For this review, take the finished solid that the model builds, in its own axes (mm). A direction names the side the tool comes from. Coordinates: 2 decimals unless noted, no trailing zeros. Write each loop counter-clockwise with the first axis right and the second up, starting at its lowest first coordinate (ties: lowest second). Pieces come first, ordered by that corner, then holes.
1) We need section A-A on y = 98.2. Write out the cut boundary in (x, z).
2) Insertion check: P1, Ø4, axis at y = 17, z = -4, coming from the -X side; P2, Ø2, axis at y = 87, z = 1.5, coming from the +X side; P3, Ø2, axis at x = -3, y = 59.5, coming from the +Z side. Each pin has a flat end and moves straight along its axis. Give the tip position at first contact, or say it passes through.
3) We need section B-B on y = 7. Write out the cut boundary in (x, z).
4) Mouldability with a two-part tool opening along Y and no side actions: class faces 3 (the face through (-4.88, 2.1, -1.08)), 4 (the face through (0.07, 97.377, -1.986)), 5 (the face through (0, 0, 0)) as pulls with the +Y half, pulls with the -Y half, needs draft (parallel to the pull), parting line crosses it, or undercut.
5) To check wall thickness, follow line 1 along Y through (x, z) = (-0.25, 0); line 2 along Y through (x, z) = (-3, -3.5); line 3 along Z through (x, y) = (-0.25, 98.2). State the ranges of each line that lie inside material, in increasing order.
6) For faces 1 (the face through (1.352, 45.944, -4.292)), 2 (the face through (-4.88, 25.02, -1.08)), list the 3-axis set-ups (+Z, -Z, +X, -X, +Y, -Y) from which the entire face can be reached by the end or side of a thin tool; tool diameter is ignored.
from build123d import *

# Parameters (mm, degrees)
SKETCH1_R            = 5
BOSS_EXTRUDE1_DEPTH  = 113.2
CUT_EXTRUDE2_START   = -4.25
SKETCH2_R            = 5
SKETCH2_R_2          = 4.5
CUT_EXTRUDE2_DEPTH   = 0.8
CUT_EXTRUDE3_START   = -45.55
SKETCH2_2_R          = 5
SKETCH2_2_R_2        = 4.5
CUT_EXTRUDE3_DEPTH   = 0.8
CUT_EXTRUDE4_START   = -50.35
SKETCH2_3_R          = 5
SKETCH2_3_R_2        = 4.5
CUT_EXTRUDE4_DEPTH   = 0.8
CUT_EXTRUDE5_START   = -91.65
SKETCH2_4_R          = 5
SKETCH2_4_R_2        = 4.5
CUT_EXTRUDE5_DEPTH   = 0.8
SKETCH4_R            = 1.5
CUT_EXTRUDE6_DEPTH   = 114.750780217
M4_CLEARANCE_HOLE1_D = 4.3


with BuildPart() as part:
    # Sketch1 → Boss-Extrude1 (new body)
    with BuildSketch(Plane(origin=(0, 0, 0), x_dir=(1, 0, 0), z_dir=(0, 1, 0))):
        with Locations(Location((0, 0, 0), (0, 0, 270))):
            Circle(SKETCH1_R)
    extrude(amount=BOSS_EXTRUDE1_DEPTH)

    # Sketch2 → Cut-Extrude2 (cut)
    with BuildSketch(Plane.XZ.offset(CUT_EXTRUDE2_START)):
        with Locations(Location((0, 0, 0), (0, 0, 270))):
            Circle(SKETCH2_R)
        with Locations(Location((0, 0, 0), (0, 0, 270))):
            Circle(SKETCH2_R_2, mode=Mode.SUBTRACT)
    extrude(amount=-CUT_EXTRUDE2_DEPTH, mode=Mode.SUBTRACT)

    # Sketch2_2 → Cut-Extrude3 (cut)
    with BuildSketch(Plane.XZ.offset(CUT_EXTRUDE3_START)):
        with Locations(Location((0, 0, 0), (0, 0, 270))):
            Circle(SKETCH2_2_R)
        with Locations(Location((0, 0, 0), (0, 0, 270))):
            Circle(SKETCH2_2_R_2, mode=Mode.SUBTRACT)
    extrude(amount=-CUT_EXTRUDE3_DEPTH, mode=Mode.SUBTRACT)

    # Sketch2_3 → Cut-Extrude4 (cut)
    with BuildSketch(Plane.XZ.offset(CUT_EXTRUDE4_START)):
        with Locations(Location((0, 0, 0), (0, 0, 270))):
            Circle(SKETCH2_3_R)
        with Locations(Location((0, 0, 0), (0, 0, 270))):
            Circle(SKETCH2_3_R_2, mode=Mode.SUBTRACT)
    extrude(amount=-CUT_EXTRUDE4_DEPTH, mode=Mode.SUBTRACT)

    # Sketch2_4 → Cut-Extrude5 (cut)
    with BuildSketch(Plane.XZ.offset(CUT_EXTRUDE5_START)):
        with Locations(Location((0, 0, 0), (0, 0, 270))):
            Circle(SKETCH2_4_R)
        with Locations(Location((0, 0, 0), (0, 0, 270))):
            Circle(SKETCH2_4_R_2, mode=Mode.SUBTRACT)
    extrude(amount=-CUT_EXTRUDE5_DEPTH, mode=Mode.SUBTRACT)

    # Sketch4 → Cut-Extrude6 (cut, through all)
    with BuildSketch(Plane(origin=(-5, 0, 0), x_dir=(0, 0, -1), z_dir=(1, 0, 0))):
        with Locations(Location((0, 98.2, 0), (0, 0, 180))):
            Circle(SKETCH4_R)
    extrude(amount=CUT_EXTRUDE6_DEPTH, mode=Mode.SUBTRACT)

    # M4 Clearance Hole1 (through all)
    with Locations(Plane.ZY.offset(5)):
        with Locations((0, 98.2)):
            Hole(M4_CLEARANCE_HOLE1_D / 2)


solid = part.part
Result:
1. outline: (-4.51, -2.15) arc R5 ccw to (4.51, -2.15) - close; (-4.51, 2.15) - (4.51, 2.15) arc R5 ccw to start
2. P1: stops at x = -4.58
2. P2: stops at x = 4.97
2. P3: stops at z = 4.58
3. outline: circle Ø10 at (0, 0)
4. face 3: needs draft
4. face 4: undercut
4. face 5: pulls with the -Y half
5. line 1: y = 0 to 96.05, 100.35 to 113.2
5. line 2: y = 0 to 4.25, 5.05 to 45.55, 46.35 to 50.35, 51.15 to 91.65, 92.45 to 113.2
5. line 3: z = -4.99 to -2.15, 2.15 to 4.99
6. face 1: none
6. face 2: +Y, -Y
